For this review, take the finished solid that the model builds, in its own axes (mm). Face numbers are marked on the shaded views. A direction names the side the tool comes from. Coordinates: 2 decimals unless noted, no trailing zeros. Order: outer loops, then holes, each group sorted by start corner. A loop starts at its lowest first (then second) coordinate and runs counter-clockwise, first axis right, second up. Notation, with made-up numbers: (-14, -11) -> (39, -11) arc R23 ccw to (39, 15) -> close; hole circle Ø5 at (-17.5, -19.5). An arc over 180 degrees is marked (long way). Return JSON: item names as keys, results as strings. Group by question number.
Item 1: For line 1 along X through (y, z) = (102, -3.5); line 2 along X through (y, z) = (94, -2); line 3 along X through (y, z) = (93, -1.5), list the stretches that pass through material, from the lowest coordinate up.
Item 2: Take a section at C-C (z = -1). Write out the cut boundary in (x, y).
Item 3: Take a section at D-D (x = 65). Write out the cut boundary in (y, z), then the cut area to 4 significant figures.
Item 4: Machinability: for the marked faces 1 and 2, which of the approach directions +Z, -Z, +X, -X, +Y, -Y give a long, thin tool a straight path to every point of the face, cutting with its end or side? Answer none if there is none.
Item 5: Draft analysis for pull direction X (two halves, no side actions). For the marked faces 3 and 4, state which applies: +X half, -X half, draft (parallel to the pull), parting line (faces both ways), or undercut.
Item 6: Insertion check: pin 1 (3 mm diameter, centred on y = 82, z = -4.5, fed in from +X); pin 2 (1 mm diameter, centred on y = 90.5, z = -3, fed in from -X); pin 3 (1.1 mm diameter, centred on y = 102.5, z = -2, fed in from -X). Each pin has a flat end and moves straight along its axis. Give the tip position at first contact, or say it passes through.
Item 7: Take a section at B-B (y = 93.75). Write out the cut boundary in (x, z).
Item 8: Take a section at A-A (y = 99.5). Write out the cut boundary in (x, z).
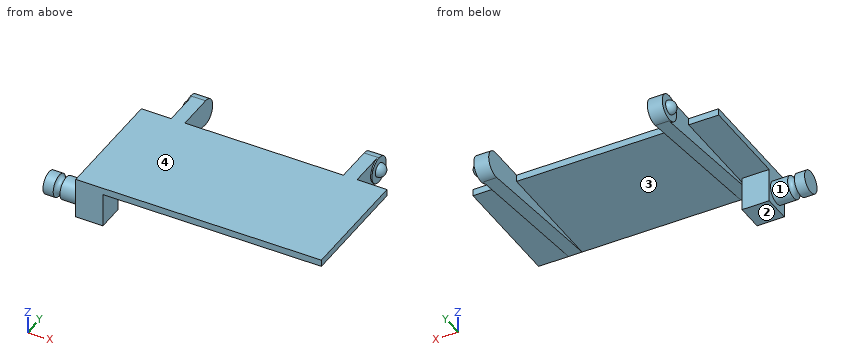
```python
from build123d import *

# Parameters (mm, degrees)
PAD038_DEPTH             = 1
PAD039_DEPTH             = 2.2
POCKET022_DEPTH          = 0.2
PAD040_DEPTH             = 2.2
POCKET023_DEPTH          = 0.2
SKETCH063_W              = 4
SKETCH063_H              = 4
PAD041_DEPTH             = 5
SKETCH064_R              = 1.65
PAD042_DEPTH             = 5
SKETCH065_R              = 0.5
PAD084_DEPTH             = 2
PAD085_DEPTH             = 2
CLONE003_PLACEMENT_ANGLE = 180


with BuildPart() as part:
    # Sketch058 (on DatumPlane) → Pad038 (new body)
    with BuildSketch(Plane(origin=(0, 0, -0.6), x_dir=(1, 0, 0), z_dir=(0, 0, -1))):
        Polygon((45.85, -61.65), (45.85, -79.1), (81.95, -79.1), (81.95, -61.65), (77.55, -61.65), (77.55, -58.65), (77.75, -58.65), (77.75, -56.15), (75.55, -56.15), (75.55, -61.65), (52.25, -61.65), (52.25, -56.15), (50.05, -56.15), (50.05, -58.65), (50.25, -58.65), (50.25, -61.65), align=None)
    extrude(amount=PAD038_DEPTH)

    # Sketch059 (on Face13 of Pad038) → Pad039 (join)
    with BuildSketch(Plane(origin=(50.05, 0, -0.6), x_dir=(0, 1, 0), z_dir=(-1, 0, 0))):
        with BuildLine():
            ThreePointArc((57.82332, 1), (55.175321, 3.530951), (56.15, 0))
            Line((56.15, 1), (56.15, 0))
            Line((57.82332, 1), (56.15, 1))
        make_face()
    extrude(amount=-PAD039_DEPTH)

    # Sketch060 (on Face18 of Pad039) → Pocket022 (cut)
    with BuildSketch(Plane(origin=(50.05, 0, -0.6), x_dir=(0, 1, 0), z_dir=(-1, 0, 0))):
        with BuildLine():
            ThreePointArc((56.15, 0), (57.124679, 0.269049), (57.82332, 1))
            Line((57.82332, 1), (58.65, 1))
            Line((58.65, 1), (58.65, 0))
            Line((58.65, 0), (56.15, 0))
        make_face()
    extrude(amount=-POCKET022_DEPTH, mode=Mode.SUBTRACT)

    # Sketch061 (on Face10 of Pocket022) → Pad040 (join)
    with BuildSketch(Plane(origin=(77.75, 0, -0.6), x_dir=(0, -1, 0), z_dir=(1, 0, 0))):
        with BuildLine():
            ThreePointArc((-56.15, 0), (-55.175321, 3.530951), (-57.82332, 1))
            Line((-57.82332, 1), (-56.15, 1))
            Line((-56.15, 1), (-56.15, 0))
        make_face()
    extrude(amount=-PAD040_DEPTH)

    # Sketch062 (on Face16 of Pad040) → Pocket023 (cut)
    with BuildSketch(Plane(origin=(77.75, 0, -0.6), x_dir=(0, -1, 0), z_dir=(1, 0, 0))):
        with BuildLine():
            ThreePointArc((-57.82332, 1), (-57.124679, 0.269049), (-56.15, 0))
            Line((-58.65, 0), (-56.15, 0))
            Line((-58.65, 1), (-58.65, 0))
            Line((-57.82332, 1), (-58.65, 1))
        make_face()
    extrude(amount=-POCKET023_DEPTH, mode=Mode.SUBTRACT)

    # Sphere004 → Sphere004 (revolve)
    with BuildSketch(Plane(origin=(50.05, 56.15, -2.5), x_dir=(0, 1, 0), z_dir=(0, 0, -1))):
        with BuildLine():
            ThreePointArc((0, -1), (1, 0), (0, 1))
            Line((0, 1), (0, -1))
        make_face()
    revolve(axis=Axis((50.05, 56.15, -2.5), (1, 0, 0)))

    # Sphere005 → Sphere005 (revolve)
    with BuildSketch(Plane(origin=(77.75, 56.15, -2.5), x_dir=(0, 1, 0), z_dir=(0, 0, -1))):
        with BuildLine():
            ThreePointArc((0, -1), (1, 0), (0, 1))
            Line((0, 1), (0, -1))
        make_face()
    revolve(axis=Axis((77.75, 56.15, -2.5), (1, 0, 0)))

    # Sketch063 (on Face5 of Sphere005) → Pad041 (join)
    with BuildSketch(Plane(origin=(77.75, 56.15, -1.6), x_dir=(0, 1, 0), z_dir=(0, 0, -1))):
        with Locations((20.95, 2.2)):
            Rectangle(SKETCH063_W, SKETCH063_H)
    extrude(amount=PAD041_DEPTH)

    # Sketch064 (on Face21 of Pad041) → Pad042 (join)
    with BuildSketch(Plane(origin=(81.95, 56.15, -2.5), x_dir=(0, 1, 0), z_dir=(1, 0, 0))):
        with Locations((20.95, -1.599996)):
            Circle(SKETCH064_R)
    extrude(amount=PAD042_DEPTH)

    # Sketch065 (on DatumPlane) → Groove002 (revolve, cut)
    with BuildSketch(Plane(origin=(84.45, 77.1, -4.1), x_dir=(0, 1, 0), z_dir=(0, 0, -1))):
        with Locations((1.680544, 0.5)):
            Circle(SKETCH065_R)
    revolve(axis=Axis((84.45, 77.1, -4.1), (1, 0, 0)), mode=Mode.SUBTRACT)

    # Sketch107 (on Face15 of Groove002) → Pad084 (join)
    with BuildSketch(Plane(origin=(52.25, 56.15, -2.5), x_dir=(0, 1, 0), z_dir=(1, 0, 0))):
        Polygon((22.95, 0.900005), (0.231255, -1.885874), (1.67332, 0.9), align=None)
    extrude(amount=-PAD084_DEPTH)

    # Sketch108 (on Face14 of Pad084) → Pad085 (join)
    with BuildSketch(Plane(origin=(75.55, 56.15, -2.5), x_dir=(0, 1, 0), z_dir=(-1, 0, 0))):
        Polygon((1.67332, -0.9), (22.95, -0.900005), (0.231255, 1.885874), align=None)
    extrude(amount=-PAD085_DEPTH)


with BuildPart() as part_1:
    # Clone003 placement: moved
    add(part.part.moved(Location((91.8, 159.4, 0))).rotate(Axis((91.8, 159.4, 0), (0, 0, -1)), CLONE003_PLACEMENT_ANGLE))


with BuildPart() as part_2:
    # Body021 placement: moved
    add(part_1.part.moved(Location((36, 0, 0))))


solid = part_2.part
```
Findings below:
{
 "1": {"line 1": "x = 50.05 to 52.25, 75.55 to 77.75", "line 2": "x = 50.25 to 52.25, 75.55 to 77.55", "line 3": "x = 45.85 to 81.95"},
 "2": {"outline": "(45.85, 80.3) -> (81.95, 80.3) -> (81.95, 97.75) -> (77.55, 97.75) -> (77.55, 102.08) -> (77.75, 102.08) -> (77.75, 104.42) -> (75.55, 104.42) -> (75.55, 97.75) -> (52.25, 97.75) -> (52.25, 104.42) -> (50.05, 104.42) -> (50.05, 102.08) -> (50.25, 102.08) -> (50.25, 97.75) -> (45.85, 97.75) -> close"},
 "3": {"outline": "(80.3, -1.6) -> (97.75, -1.6) -> (97.75, -0.6) -> (80.3, -0.6) -> close", "area": "17.45 mm2"},
 "4": {"face 1": "-X", "face 2": "-Z, +X, -X, +Y, -Y"},
 "5": {"face 3": "undercut", "face 4": "draft"},
 "6": {"pin 1": "stops at x = 49.85", "pin 2": "stops at x = 50.25", "pin 3": "stops at x = 49.11"},
 "7": {"outline": "(45.85, -1.6) -> (50.25, -1.6) -> (50.25, -3.25) -> (52.25, -3.25) -> (52.25, -1.6) -> (75.55, -1.6) -> (75.55, -3.25) -> (77.55, -3.25) -> (77.55, -1.6) -> (81.95, -1.6) -> (81.95, -0.6) -> (45.85, -0.6) -> close"},
 "8": {"outline": "(50.25, -3.95) -> (52.25, -3.95) -> (52.25, -0.6) -> (50.25, -0.6) -> close; (75.55, -3.95) -> (77.55, -3.95) -> (77.55, -0.6) -> (75.55, -0.6) -> close"}
}
